from build123d import *

# Parameters (mm, degrees)
SKETCH_1_R      = 2
EXTRUDE_1_DEPTH = 22


with BuildPart() as part:
    # 草图1 → 凸台-拉伸1 (new body)
    with BuildSketch(Plane(origin=(0, 0, 0), x_dir=(1, 0, 0), z_dir=(0, 1, 0))):
        Polygon((0, 0), (0, 34), (30, 34), (30, 19), (41, 19), (41, 34), (71, 34), (71, 0), (41, 0), (41, 15), (30, 15), (30, 0), align=None)
        with Locations(Location((6, 29, 0), (0, 0, 270))):
            Circle(SKETCH_1_R, mode=Mode.SUBTRACT)
        with Locations(Location((24, 29, 0), (0, 0, 90))):
            Circle(SKETCH_1_R, mode=Mode.SUBTRACT)
        with Locations(Location((24, 5, 0), (0, 0, 270))):
            Circle(SKETCH_1_R, mode=Mode.SUBTRACT)
        with Locations(Location((6, 5, 0), (0, 0, 90))):
            Circle(SKETCH_1_R, mode=Mode.SUBTRACT)
        with Locations(Location((47, 29, 0), (0, 0, 270))):
            Circle(SKETCH_1_R, mode=Mode.SUBTRACT)
        with Locations(Location((47, 5, 0), (0, 0, 90))):
            Circle(SKETCH_1_R, mode=Mode.SUBTRACT)
        with Locations(Location((65, 5, 0), (0, 0, 270))):
            Circle(SKETCH_1_R, mode=Mode.SUBTRACT)
        with Locations(Location((65, 29, 0), (0, 0, 90))):
            Circle(SKETCH_1_R, mode=Mode.SUBTRACT)
    extrude(amount=EXTRUDE_1_DEPTH)


solid = part.part
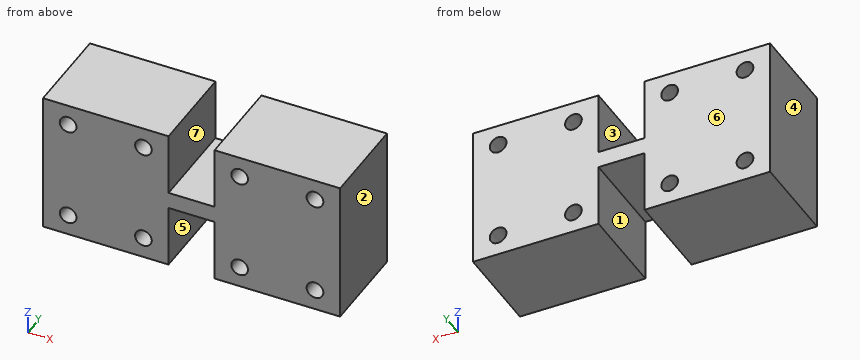
Design review of the part built by this model. Coordinates are the model's own, in mm. Face numbers are marked on the shaded views. A direction names the side the tool comes from. Round coordinates to 2 decimals unless told otherwise and drop trailing zeros. Write each loop counter-clockwise with the first axis right and the second up, starting at its lowest first coordinate (ties: lowest second). Pieces come first, ordered by that corner, then holes.
Item 1: Consider section D-D on z = -29. Give the boundary of the cut face in (x, y).
Item 2: For the marked faces 1, 2 and 3, list the 3-axis set-ups (+Z, -Z, +X, -X, +Y, -Y) from which the entire face can be reached by the end or side of a thin tool; tool diameter is ignored.
Item 3: For pin 1 Ø5 at (x, z) = (24, -5) entering from +Y; pin 2 Ø3 at (x, z) = (65, -5) entering from +Y; pin 3 Ø3.5 at (x, y) = (38, 7) entering from -Z; pin 4 Ø9 at (x, y) = (35.5, 6.5) entering from +Z, all flat-tipped, find the tip position at first contact; note any pin that passes through.
Item 4: Consider section B-B on x = 47. Give the boundary of the cut face in (y, z).
Item 5: Consider section A-A on z = -2. Give the boundary of the cut face in (x, y).
Item 6: Draft analysis for pull direction X (two halves, no side actions). For the marked faces 4, 5, 6 and 7, state which applies: released by +X, released by -X, zero draft, split by the parting line, or undercut.
Item 7: Wall thickness on L1, parallel to X at y = 9.25, z = -29; L2, parallel to Z at x = 48, y = 13; L3, parallel to X at y = 20, z = -10.5: over which ranges is each line inside the solid? List them lowest first.
Item 8: Consider section C-C on y = 6.75. Count the separate pieces of the cut face and the enclosed holes in it, and give its area (3 significant figures).
Check values:
1. outline: (0, 0) - (4, 0) - (4, 22) - (0, 22) - close; (8, 0) - (22, 0) - (22, 22) - (8, 22) - close; (26, 0) - (30, 0) - (30, 22) - (26, 22) - close; (41, 0) - (45, 0) - (45, 22) - (41, 22) - close; (49, 0) - (63, 0) - (63, 22) - (49, 22) - close; (67, 0) - (71, 0) - (71, 22) - (67, 22) - close
2. face 1: -Z, +Y, -Y
2. face 2: +Z, -Z, +X, +Y, -Y
2. face 3: +Z, +Y, -Y
3. pin 1: stops at y = 22
3. pin 2: passes through
3. pin 3: stops at z = -19
3. pin 4: stops at z = -15
4. outline: (0, -34) - (22, -34) - (22, -31) - (0, -31) - close; (0, -27) - (22, -27) - (22, -7) - (0, -7) - close; (0, -3) - (22, -3) - (22, 0) - (0, 0) - close
5. outline: (0, 0) - (30, 0) - (30, 22) - (0, 22) - close; (41, 0) - (71, 0) - (71, 22) - (41, 22) - close
6. face 4: released by -X
6. face 5: undercut
6. face 6: zero draft
6. face 7: undercut
7. L1: x = 0 to 4, 8 to 22, 26 to 30, 41 to 45, 49 to 63, 67 to 71
7. L2: z = -34 to -30.73, -27.27 to -6.73, -3.27 to 0
7. L3: x = 0 to 30, 41 to 71
8. separate pieces: 1
8. enclosed holes: 8
8. area: 1,980 mm2
